```python
from build123d import *

# Parameters (mm, degrees)
SKETCH1_R           = 92.075
SKETCH1_R_2         = 88.9
BOSS_EXTRUDE1_DEPTH = 374.65
SKETCH2_W           = 177.8
SKETCH2_H           = 254
CUT_EXTRUDE1_DEPTH  = 93.075


with BuildPart() as part:
    # Sketch1 → Boss-Extrude1 (new body)
    with BuildSketch(Plane(origin=(0, 0, 0), x_dir=(1, 0, 0), z_dir=(0, 1, 0))):
        Circle(SKETCH1_R)
        Circle(SKETCH1_R_2, mode=Mode.SUBTRACT)
    extrude(amount=BOSS_EXTRUDE1_DEPTH)

    # Sketch2 → Cut-Extrude1 (cut, through all)
    with BuildSketch(Plane.XY):
        with Locations((0, 187.325)):
            Rectangle(SKETCH2_W, SKETCH2_H)
    extrude(amount=CUT_EXTRUDE1_DEPTH, mode=Mode.SUBTRACT)


solid = part.part
```
Work out the finished part from the listing and answer in its coordinate system (mm). A direction names the side the tool comes from. Round coordinates to 2 decimals unless told otherwise and drop trailing zeros. Write each loop counter-clockwise with the first axis right and the second up, starting at its lowest first coordinate (ties: lowest second). Pieces come first, ordered by that corner, then holes.
1) Flat-ended cylindrical pins translate along their axes: P1, Ø12, axis at x = 59.5, y = 289.5, coming from the -Z side; P2, Ø5, axis at x = -39, y = 54, coming from the -Z side; P3, Ø12, axis at x = 37.5, y = 161.5, coming from the +Z side. Find the tip coordinate at first contact, or state that the pin passes through.
2) Which of the six approach directions +Z, -Z, +X, -X, +Y, -Y give full straight-line access (tool end or side, diameter ignored) to faces 1 (the face through (-75.5, 374.65, -48.2)), 2 (the face through (88.9, 186, 12))?
3) Consider probe 1 along Y at (x, z) = (64.5, 65.5) (3 decimals); probe 2 along X at (y, z) = (134.5, 0) (3 decimals); probe 3 along Z at (x, y) = (40, 332.5). Determine where each line is inside the solid, lowest interval first.
4) Determine the mould class of faces 3 (the face through (-11.99, 184.7, -91.29)), 4 (the face through (-75.5, 0, -48.2)), 5 (the face through (-11.573, 184.702, -88.143)) for opening direction X: pulls with the +X half, pulls with the -X half, needs draft (parallel to the pull), parting line crosses it, or undercut.
5) A cutting plane is placed at C-C on y = 23. Determine the outline of the cut face in (x, z) (3 decimals).
6) A cutting plane is placed at D-D on z = 62. Determine the outline of the cut face in (x, y) (3 decimals), and give its area (3 significant figures).
7) A cutting plane is placed at A-A on x = 0. Determine the outline of the cut face in (y, z) (3 decimals), and give its area (3 significant figures).
8) A cutting plane is placed at B-B on z = -67.5. Determine the outline of the cut face in (x, y).
Entries:
1. P1: stops at z = -74.94
1. P2: stops at z = -84.53
1. P3: stops at z = -77.53
2. face 1: +Z, -Z, +X, -X, +Y
2. face 2: +Z
3. probe 1: y = 0 to 60.325, 314.325 to 374.65
3. probe 2: x = -92.075 to -88.9, 88.9 to 92.075
3. probe 3: z = -82.93 to -79.39, 79.39 to 82.93
4. face 3: parting line crosses it
4. face 4: needs draft
4. face 5: undercut
5. outline: circle Ø184.15 at (0, 0); hole circle Ø177.8 at (0, 0)
6. outline: (-68.072, 0) - (-63.712, 0) - (-63.712, 60.325) - (-68.072, 60.325) - close; (-68.072, 314.325) - (-63.712, 314.325) - (-63.712, 374.65) - (-68.072, 374.65) - close; (63.712, 0) - (68.072, 0) - (68.072, 60.325) - (63.712, 60.325) - close; (63.712, 314.325) - (68.072, 314.325) - (68.072, 374.65) - (63.712, 374.65) - close
6. area: 1,050 mm2
7. outline: (0, -92.075) - (374.65, -92.075) - (374.65, -88.9) - (0, -88.9) - close; (0, 88.9) - (60.325, 88.9) - (60.325, 92.075) - (0, 92.075) - close; (314.325, 88.9) - (374.65, 88.9) - (374.65, 92.075) - (314.325, 92.075) - close
7. area: 1,570 mm2
8. outline: (-62.62, 0) - (-57.85, 0) - (-57.85, 374.65) - (-62.62, 374.65) - close; (57.85, 0) - (62.62, 0) - (62.62, 374.65) - (57.85, 374.65) - close
